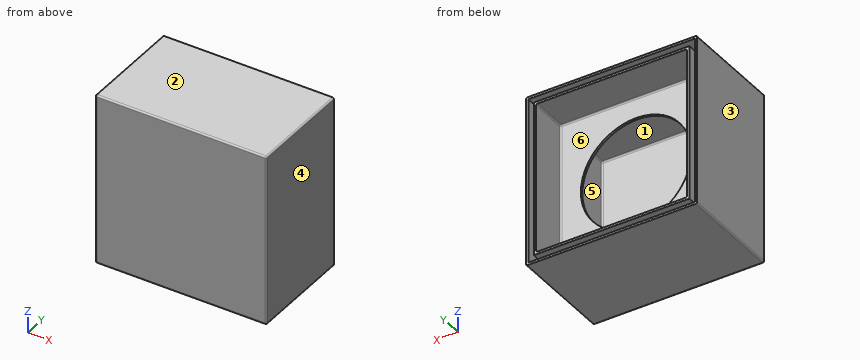
```python
from build123d import *

# Parameters (mm, degrees)
SKETCH1_W             = 200
SKETCH1_H             = 200
SKETCH1_W_2           = 194
SKETCH1_H_2           = 194
BOSS_EXTRUDE1_DEPTH   = 132
SKETCH1_W_3           = 220
SKETCH1_H_3           = 220
SKETCH1_W_4           = 214
SKETCH1_H_4           = 214
BOSS_EXTRUDE1_2_DEPTH = 132
SKETCH3_W             = 220
SKETCH3_H             = 220
BOSS_EXTRUDE3_DEPTH   = 3
SKETCH4_W             = 194
SKETCH4_H             = 194
BOSS_EXTRUDE4_DEPTH   = 3
SKETCH5_R             = 71
CUT_EXTRUDE1_DEPTH    = 3
SKETCH7_R             = 8.5
CUT_EXTRUDE3_DEPTH    = 3
FILLET1_R             = 2


with BuildPart() as part:
    # Sketch1 → Boss-Extrude1 (new body)
    with BuildSketch(Plane(origin=(0, 0, 0), x_dir=(1, 0, 0), z_dir=(0, 1, 0))):
        Rectangle(SKETCH1_W, SKETCH1_H)
        Rectangle(SKETCH1_W_2, SKETCH1_H_2, mode=Mode.SUBTRACT)
    extrude(amount=BOSS_EXTRUDE1_DEPTH)



with BuildPart() as body_2:
    # Sketch1 → Boss-Extrude1 2 (new body)
    with BuildSketch(Plane(origin=(0, 0, 0), x_dir=(1, 0, 0), z_dir=(0, 1, 0))):
        Rectangle(SKETCH1_W_3, SKETCH1_H_3)
        Rectangle(SKETCH1_W_4, SKETCH1_H_4, mode=Mode.SUBTRACT)
    extrude(amount=BOSS_EXTRUDE1_2_DEPTH)


with BuildPart() as part_1:
    add(part.part)

    add(body_2.part)  # Boss-Extrude3 merges body 2
    # Sketch3 → Boss-Extrude3 (add)
    with BuildSketch(Plane.XZ):
        Rectangle(SKETCH3_W, SKETCH3_H)
    extrude(amount=BOSS_EXTRUDE3_DEPTH)

    # Sketch4 → Boss-Extrude4 (add)
    with BuildSketch(Plane(origin=(0, 80, 0), x_dir=(1, 0, 0), z_dir=(0, 1, 0))):
        Rectangle(SKETCH4_W, SKETCH4_H)
    extrude(amount=BOSS_EXTRUDE4_DEPTH)

    # Sketch5 → Cut-Extrude1 (cut)
    with BuildSketch(Plane(origin=(0, 83, 0), x_dir=(1, 0, 0), z_dir=(0, 1, 0))):
        with Locations(Location((0, 0, 0), (0, 0, 270))):
            Circle(SKETCH5_R)
    extrude(amount=-CUT_EXTRUDE1_DEPTH, mode=Mode.SUBTRACT)

    # Sketch7 → Cut-Extrude3 (cut)
    with BuildSketch(Plane(origin=(0, 83, 0), x_dir=(1, 0, 0), z_dir=(0, 1, 0))):
        with Locations(Location((-77, 77, 0), (0, 0, 270))):
            Circle(SKETCH7_R)
    extrude(amount=-CUT_EXTRUDE3_DEPTH, mode=Mode.SUBTRACT)

    # Fillet1
    fillet1_edges = [part_1.edges().sort_by_distance(p)[0] for p in [
        (-97, 0, 0),
        (0, 0, 97),
        (97, 0, 0),
        (0, 0, -97),
        (-97, 107.5, -97),
        (-97, 107.5, 97),
        (97, 107.5, 97),
        (97, 107.5, -97),
        (110, 64.5, -110),
        (110, 64.5, 110),
        (-110, 64.5, 110),
        (-110, 64.5, -110),
        (110, -3, 0),
        (0, -3, 110),
        (-110, -3, 0),
        (0, -3, -110),
        (-97, 40, -97),
        (-97, 40, 97),
        (97, 40, 97),
        (97, 40, -97),
        (97, 83, 0),
        (0, 83, -97),
        (-97, 83, 0),
        (0, 83, 97),
    ]]
    fillet(fillet1_edges, radius=FILLET1_R)


solid = part_1.part
```
The model under review builds one solid part; all positions refer to its coordinate system, in mm. Face numbers are marked on the shaded views. A direction names the side the tool comes from. Round coordinates to 2 decimals unless told otherwise and drop trailing zeros. Loops run counter-clockwise (first coordinate to the right, second up) from the corner with the lowest first, then second, coordinate; pieces in that order, holes last. Notation, with made-up numbers: (-11, -35.5) - (1, -35.5) arc R18 ccw to (1, -24.5) - close; hole circle Ø10 at (23, 45). An arc over 180 degrees is marked (long way). Use a Markdown table: item, result. Add a question column.
Q1. For probe 1 along X at (y, z) = (29.5, 91.5); probe 2 along X at (y, z) = (80.75, -77), list the stretches that pass through material, from the lowest coordinate up.
Q2. Add section A-A (z = -92). State the section outline as (x, y) points.
Q3. Add section C-C (x = 91.5). State the section outline as (y, z) points, plus the area to 3 significant figures.
Q4. Machinability: for the marked faces 4, 5 and 6, which of the approach directions +Z, -Z, +X, -X, +Y, -Y give a long, thin tool a straight path to every point of the face, cutting with its end or side? Answer none if there is none.
Q5. The part is to be moulded in two halves that separate along X. For the marked faces 1, 2 and 3, say which applies: pulls with the +X half, pulls with the -X half, needs draft (parallel to the pull), parting line crosses it, or undercut.
Q6. Insertion check: pin 1 Ø5 at (x, z) = (-43, -38.5) entering from +Y; pin 2 Ø3 at (x, z) = (40, -69.5) entering from +Y. Each pin has a flat end and moves straight along its axis. Give the tip position at first contact, or say it passes through.
Worked answers:
| question | item | result |
|---|---|---|
| 1 | probe 1 | -110 to -107, -100 to -97, 97 to 100, 107 to 110 |
| 1 | probe 2 | -110 to -107, -100 to -85.5, -68.5 to 100, 107 to 110 |
| 2 | outline | (-110, -1) arc R2 ccw to (-108, -3) - (108, -3) arc R2 ccw to (110, -1) - (110, 132) - (107, 132) - (107, 0) - (100, 0) - (100, 132) - (97, 132) - (97, 85) arc R2 cw to (95, 83) - (-95, 83) arc R2 cw to (-97, 85) - (-97, 132) - (-100, 132) - (-100, 0) - (-107, 0) - (-107, 132) - (-110, 132) - close; hole (-97, 2) arc R2 ccw to (-95, 0) - (95, 0) arc R2 ccw to (97, 2) - (97, 80) - (-97, 80) - close |
| 3 | outline | (-3, -108) arc R2 ccw to (-1, -110) - (132, -110) - (132, -107) - (0, -107) - (0, -100) - (132, -100) - (132, -97) - (85, -97) arc R2 cw to (83, -95) - (83, 95) arc R2 cw to (85, 97) - (132, 97) - (132, 100) - (0, 100) - (0, 107) - (132, 107) - (132, 110) - (-1, 110) arc R2 ccw to (-3, 108) - close; hole (0, -95) arc R2 ccw to (2, -97) - (80, -97) - (80, 97) - (2, 97) arc R2 ccw to (0, 95) - close |
| 3 | area | 2,830 mm² |
| 4 | face 4 | +Z, -Z, +X, +Y, -Y |
| 4 | face 5 | none |
| 4 | face 6 | +Y |
| 5 | face 1 | undercut |
| 5 | face 2 | needs draft |
| 5 | face 3 | pulls with the -X half |
| 6 | pin 1 | y = 0 |
| 6 | pin 2 | y = 83 |
